Geometry check sheet. Reference: the model listing, model coordinates, mm. A direction names the side the tool comes from. Give positions to 0.01 mm unless a question says otherwise; leave off trailing zeros. Order: outer loops, then holes, each group sorted by start corner. A loop starts at its lowest first (then second) coordinate and runs counter-clockwise, first axis right, second up. Notation, with made-up numbers: M -17.5,72 L -8.5,72 A16 ccw -8.5,86 Z; hole C -30.5,48.5 d5. An arc over 180 degrees is marked long. Answer as CSV lines item,"result". Start each with the question number.
Q1. Section check B-B, the plane x = 0. Record the boundary of the cut face in (y, z), then the cut area to 3 significant figures.
Q2. Section check A-A, the plane y = 0. Record the boundary of the cut face in (x, z).
Q3. Section check C-C, the plane z = 13.5. Record the boundary of the cut face in (x, y), then the cut area to 3 significant figures.
Q4. Go/stop test with flat-tipped pins: pin 1 (5.5 mm diameter, centred on x = 4, y = 4.5, fed in from -Z); pin 2 (0.6 mm diameter, centred on x = -12.5, y = -7, fed in from -Z); pin 3 (2.5 mm diameter, centred on x = 12.25, y = -7.08, fed in from -Z). Record where each tip stops, or that it passes through.
Q5. Thickness scan on line 1 (Y direction, x = 0, z = -2.05); line 2 (Z direction, x = -13, y = 7); line 3 (Y direction, x = 0.5, z = 2.5). Record the ranges inside material, lowest first.
Q6. Mould release check, pull along X, two halves, no side actions. Record for faces 1 (the cylindrical face through (11.275, -6.767, 3.352)), 2 (the cylindrical face through (2.17, -9.76, -2.07)), 3 (the flat face through (-1, 8, -4.7)): +X half, -X half, draft (parallel to the pull), parting line (faces both ways), or undercut.
Q7. Set-up check for faces 4 (the flat face through (-14, -3, 6.8)), 5 (the flat face through (0, 0, -16.7)): record each of +Z, -Z, +X, -X, +Y, -Y from which the full face is reachable in a straight line by a thin tool's end or side.
```python
from build123d import *

# Parameters (mm, degrees)
SKETCH1_R           = 19.15
BOSS_EXTRUDE1_DEPTH = 35.3
SKETCH2_R           = 10
SKETCH2_R_2         = 7.5
BOSS_EXTRUDE2_DEPTH = 4.7
SKETCH3_R           = 3
BOSS_EXTRUDE3_DEPTH = 16.7
SKETCH4_R           = 1.008522138
SKETCH4_R_2         = 1.026344308
CUT_EXTRUDE1_DEPTH  = 6.8
FILLET1_R           = 1.5
FILLET2_R           = 0.5
FILLET3_R           = 0.5
FILLET4_R           = 0.5


with BuildPart() as part:
    # Sketch1 → Boss-Extrude1 (new body)
    with BuildSketch(Plane.XY):
        Circle(SKETCH1_R)
    extrude(amount=BOSS_EXTRUDE1_DEPTH)

    # Sketch2 → Boss-Extrude2 (add)
    with BuildSketch(Plane(origin=(0, 0, 0), x_dir=(-1, 0, 0), z_dir=(0, 0, -1))):
        Circle(SKETCH2_R)
        Circle(SKETCH2_R_2, mode=Mode.SUBTRACT)
    extrude(amount=BOSS_EXTRUDE2_DEPTH)

    # Sketch3 → Boss-Extrude3 (add)
    with BuildSketch(Plane(origin=(0, 0, 0), x_dir=(-1, 0, 0), z_dir=(0, 0, -1))):
        Circle(SKETCH3_R)
    extrude(amount=BOSS_EXTRUDE3_DEPTH)

    # Sketch4 → Cut-Extrude1 (cut)
    with BuildSketch(Plane(origin=(0, 0, 0), x_dir=(-1, 0, 0), z_dir=(0, 0, -1))):
        with Locations((-3.959842876, 13.584628975)):
            Circle(SKETCH4_R)
        with Locations((0, 14.15)):
            Circle(SKETCH4_R_2)
        with Locations((12.254259464, -7.075)):
            Circle(SKETCH4_R_2)
        with Locations((13.744555232, -3.362989962)):
            Circle(SKETCH4_R)
        with Locations((-12.254259464, -7.075)):
            Circle(SKETCH4_R_2)
        with Locations((-9.784712355, -10.221639013)):
            Circle(SKETCH4_R)
    extrude(amount=-CUT_EXTRUDE1_DEPTH, mode=Mode.SUBTRACT)

    # Fillet1
    fillet1_edges = [part.edges().sort_by_distance(p)[0] for p in [
        (-19.15, 0, 35.3),
    ]]
    fillet(fillet1_edges, radius=FILLET1_R)

    # Fillet2
    fillet2_edges = [part.edges().sort_by_distance(p)[0] for p in [
        (3, 0, -16.7),
    ]]
    fillet(fillet2_edges, radius=FILLET2_R)

    # Fillet3
    fillet3_edges = [part.edges().sort_by_distance(p)[0] for p in [
        (10, 0, -4.7),
    ]]
    fillet(fillet3_edges, radius=FILLET3_R)

    # Fillet4
    fillet4_edges = [part.edges().sort_by_distance(p)[0] for p in [
        (-19.15, 0, 0),
    ]]
    fillet(fillet4_edges, radius=FILLET4_R)


solid = part.part
```
Answer block:
1,outline,"M -19.15,0.5 A0.5 ccw -18.65,0 L -10,0 L -10,-4.2 A0.5 ccw -9.5,-4.7 L -7.5,-4.7 L -7.5,0 L -3,0 L -3,-16.2 A0.5 ccw -2.5,-16.7 L 2.5,-16.7 A0.5 ccw 3,-16.2 L 3,0 L 7.5,0 L 7.5,-4.7 L 9.5,-4.7 A0.5 ccw 10,-4.2 L 10,0 L 13.12,0 L 13.12,6.8 L 15.18,6.8 L 15.18,0 L 18.65,0 A0.5 ccw 19.15,0.5 L 19.15,33.8 A1.5 ccw 17.65,35.3 L -17.65,35.3 A1.5 ccw -19.15,33.8 Z"
1,area,"1,460 mm2"
2,outline,"M -19.15,0.5 A0.5 ccw -18.65,0 L -10,0 L -10,-4.2 A0.5 ccw -9.5,-4.7 L -7.5,-4.7 L -7.5,0 L -3,0 L -3,-16.2 A0.5 ccw -2.5,-16.7 L 2.5,-16.7 A0.5 ccw 3,-16.2 L 3,0 L 7.5,0 L 7.5,-4.7 L 9.5,-4.7 A0.5 ccw 10,-4.2 L 10,0 L 18.65,0 A0.5 ccw 19.15,0.5 L 19.15,33.8 A1.5 ccw 17.65,35.3 L -17.65,35.3 A1.5 ccw -19.15,33.8 Z"
3,outline,"C 0,0 d38.3"
3,area,"1,150 mm2"
4,pin 1,"stops at z = -4.7"
4,pin 2,"stops at z = 6.8"
4,pin 3,"stops at z = 0"
5,line 1,"y = -10 to -7.5, -3 to 3, 7.5 to 10"
5,line 2,"z = 0 to 35.3"
5,line 3,"y = -19.14 to 13.25, 15.05 to 19.14"
6,face 1,"undercut"
6,face 2,"parting line"
6,face 3,"draft"
7,face 4,"-Z"
7,face 5,"-Z, +X, -X, +Y, -Y"
